Check sheet for the modelled part. Datum: model origin and axes. Units: mm. A direction names the side the tool comes from. Coordinates: 2 decimals unless noted, no trailing zeros. Loops run counter-clockwise (first coordinate to the right, second up) from the corner with the lowest first, then second, coordinate; pieces in that order, holes last. Notation, with made-up numbers: (74, -22) -> (123, -22) arc R16 cw to (123, -18) -> close; hole circle Ø4 at (-16.5, -9.75). An arc over 180 degrees is marked (long way). Use one line per item in the form item = value.
from build123d import *

# Parameters (mm, degrees)
ESBO_O1_R                = 2
ESBO_O1_R_2              = 12
ESBO_O1_W                = 46
ESBO_O1_H                = 6
ESBO_O1_H_2              = 3
RESSALTO_EXTRUS_O1_DEPTH = 3
ESBO_O1_3_W              = 46
ESBO_O1_3_H              = 3
RESSALTO_EXTRUS_O2_DEPTH = 15
ESBO_O2_R                = 2.25
ESBO_O2_R_2              = 1.5
CORTE_EXTRUS_O1_DEPTH    = 1.5
ESBO_O2_4_R              = 1.5
CORTE_EXTRUS_O3_DEPTH    = 61.580524923
RESSALTO_EXTRUS_O3_DEPTH = 2
RESSALTO_EXTRUS_O4_DEPTH = 2
CORTE_EXTRUS_O4_START    = -2
ESBO_O7_R                = 1.5
CORTE_EXTRUS_O4_DEPTH    = 2


with BuildPart() as part:
    # Esboço1 → Ressalto-extrusão1 (new body)
    # profile 1 of 4: a face of its own
    with BuildSketch(Plane.XY):
        Polygon((-23, -2), (-23, -23), (23, -23), (23, -2), (21, -2), (21, 19), (-21, 19), (-21, -2), align=None)
        with Locations((-15.731654435, -15.268345565)):
            Circle(ESBO_O1_R, mode=Mode.SUBTRACT)
        with Locations((15.26769418, -15.067384206)):
            Circle(ESBO_O1_R, mode=Mode.SUBTRACT)
        with Locations((-15.731654435, 15.731654435)):
            Circle(ESBO_O1_R, mode=Mode.SUBTRACT)
        Circle(ESBO_O1_R_2, mode=Mode.SUBTRACT)
        with Locations((15.404994987, 15.932311736)):
            Circle(ESBO_O1_R, mode=Mode.SUBTRACT)
    # profile 2 of 4: a face of its own
    with BuildSketch(Plane.XY):
        Polygon((23, -23), (-23, -23), (-23, -25), (-23, -26), (23, -26), (23, -25), align=None)
    # profile 3 of 4: a face of its own
    with BuildSketch(Plane.XY):
        with Locations((0, -29)):
            Rectangle(ESBO_O1_W, ESBO_O1_H)
    # profile 4 of 4: a face of its own
    with BuildSketch(Plane.XY):
        with Locations((0, -33.5)):
            Rectangle(ESBO_O1_W, ESBO_O1_H_2)
    extrude(amount=RESSALTO_EXTRUS_O1_DEPTH)

    # Esboço1<3> → Ressalto-extrusão2 (add)
    with BuildSketch(Plane.XY):
        Polygon((23, -23), (-23, -23), (-23, -25), (-23, -26), (23, -26), (23, -25), align=None)
        with Locations((0, -33.5)):
            Rectangle(ESBO_O1_3_W, ESBO_O1_3_H)
    extrude(amount=-RESSALTO_EXTRUS_O2_DEPTH)

    # Esboço2 → Corte-extrusão1 (cut)
    # profile 1 of 2: a face of its own
    with BuildSketch(Plane.XZ.offset(35)):
        with Locations(Location((-18, -9.5, 0), (0, 0, 270))):
            Circle(ESBO_O2_R)
        with Locations(Location((-18, -9.5, 0), (0, 0, 270))):
            Circle(ESBO_O2_R_2, mode=Mode.SUBTRACT)
    # profile 2 of 2: a face of its own
    with BuildSketch(Plane.XZ.offset(35)):
        with Locations(Location((18, -9.5, 0), (0, 0, 270))):
            Circle(ESBO_O2_R)
        with Locations(Location((18, -9.5, 0), (0, 0, 270))):
            Circle(ESBO_O2_R_2, mode=Mode.SUBTRACT)
    extrude(amount=-CORTE_EXTRUS_O1_DEPTH, mode=Mode.SUBTRACT)

    # Esboço2<4> → Corte-extrusão3 (cut, through all)
    with BuildSketch(Plane.XZ.offset(35)):
        with Locations(Location((-18, -9.5, 0), (0, 0, 270))):
            Circle(ESBO_O2_4_R)
        with Locations(Location((18, -9.5, 0), (0, 0, 270))):
            Circle(ESBO_O2_4_R)
    extrude(amount=-CORTE_EXTRUS_O3_DEPTH, mode=Mode.SUBTRACT)

    # Esboço5 → Ressalto-extrusão3 (add)
    with BuildSketch(Plane(origin=(23, 0, 0), x_dir=(0, 0, -1), z_dir=(1, 0, 0))):
        Polygon((15, -23), (0, -6.455375179), (0, -23), align=None)
    extrude(amount=-RESSALTO_EXTRUS_O3_DEPTH)

    # Esboço6 → Ressalto-extrusão4 (add)
    with BuildSketch(Plane.ZY.offset(23)):
        Polygon((-15, -23), (0, -23), (0, -6.455375179), align=None)
    extrude(amount=-RESSALTO_EXTRUS_O4_DEPTH)

    # Esboço7 → Corte-extrusão4 (cut)
    # profile 1 of 2: a face of its own
    with BuildSketch(Plane(origin=(0, -23, 0), x_dir=(1, 0, 0), z_dir=(0, 1, 0)).offset(CORTE_EXTRUS_O4_START)):
        Polygon((-20.632829264, 7.724741314), (-17.778995512, 6.332273631), (-15.146166248, 8.107532317), (-15.367170736, 11.275258686), (-18.221004488, 12.667726369), (-20.853833752, 10.892467683), align=None)
        with Locations((-18, 9.5)):
            Circle(ESBO_O7_R, mode=Mode.SUBTRACT)
    # profile 2 of 2: a face of its own
    with BuildSketch(Plane(origin=(0, -23, 0), x_dir=(1, 0, 0), z_dir=(0, 1, 0)).offset(CORTE_EXTRUS_O4_START)):
        Polygon((17.778995512, 6.332273631), (15.146166248, 8.107532317), (15.367170736, 11.275258686), (18.221004488, 12.667726369), (20.853833752, 10.892467683), (20.632829264, 7.724741314), align=None)
        with Locations((18, 9.5)):
            Circle(ESBO_O7_R, mode=Mode.SUBTRACT)
    extrude(amount=CORTE_EXTRUS_O4_DEPTH, mode=Mode.SUBTRACT)


solid = part.part
(1) Mould release check, pull along X, two halves, no side actions. Record for faces 6 (the flat face through (0, -14, 3)), 7 (the flat face through (-21, -18, -4)), 8 (the flat face through (21, 8, 1)): +X half, -X half, draft (parallel to the pull), parting line (faces both ways), or undercut.
Established:
face_6 = draft
face_7 = undercut
face_8 = +X half
(2) Tool access check on faces 1 (the flat face through (16.77, -24.01, -11.96)), 2 (the cylindrical face through (-16.17, -17.22, 1.48)), 3 (the flat face through (21, -18, -4)), 4 (the flat face through (19, -33.5, -11)), 5 (the flat face through (0, -32, -7)). Record the directions out of +Z, -Z, +X, -X, +Y, -Y that give a thin tool (end or side, any length) a straight path to the whole face; none if there is none.
Established:
face_1 = +Y
face_2 = +Z, -Z
face_3 = -Z, +Y
face_4 = -Y
face_5 = -Z, +X, -X
(3) Section check D-D, the plane x = 7. Record the boundary of the cut face in (y, z), plus the area to 3 significant figures.
Established:
outline = (-35, -15) -> (-32, -15) -> (-32, 0) -> (-26, 0) -> (-26, -15) -> (-23, -15) -> (-23, 0) -> (-9.75, 0) -> (-9.75, 3) -> (-35, 3) -> close; (9.75, 0) -> (19, 0) -> (19, 3) -> (9.75, 3) -> close
area = 194 mm²
(4) Scan lines: line 1 along X through (y, z) = (-25.45, -9.5); line 2 along X through (y, z) = (-18, -5.25); line 3 along Y through (x, z) = (16.5, -4.25). Record each from-to range of solid material in increasing order.
Established:
line_1 = -23 to -19.5, -16.5 to 16.5, 19.5 to 23
line_2 = -23 to -21, 21 to 23
line_3 = -35 to -32, -26 to -23
(5) Section check C-C, the plane z = -2.5. Record the boundary of the cut face in (x, y), plus the area to 3 significant figures.
Established:
outline = (-23, -35) -> (23, -35) -> (23, -32) -> (-23, -32) -> close; (-23, -26) -> (23, -26) -> (23, -9.21) -> (21, -9.21) -> (21, -23) -> (-21, -23) -> (-21, -9.21) -> (-23, -9.21) -> close
area = 331 mm²
(6) Go/stop test with flat-tipped pins: P1, Ø4, axis at x = 18, z = -9.5, coming from the -Y side; P2, Ø6.5, axis at x = -17.5, z = -10, coming from the +Y side; P3, Ø3.5, axis at x = 18, z = -9.5, coming from the +Y side; P4, Ø12, axis at x = 3.5, y = -29.5, coming from the -Z side. Record where each tip stops, or that it passes through.
Established:
P1 = -33.5
P2 = -23
P3 = -25
P4 = -15
(7) Section check B-B, the plane y = 0. Record the boundary of the cut face in (x, z), plus the area to 3 significant figures.
Established:
outline = (-21, 0) -> (-12, 0) -> (-12, 3) -> (-21, 3) -> close; (12, 0) -> (21, 0) -> (21, 3) -> (12, 3) -> close
area = 54.0 mm²
(8) Section check A-A, the plane x = 0. Record the boundary of the cut face in (y, z).
Established:
outline = (-35, -15) -> (-32, -15) -> (-32, 0) -> (-26, 0) -> (-26, -15) -> (-23, -15) -> (-23, 0) -> (-12, 0) -> (-12, 3) -> (-35, 3) -> close; (12, 0) -> (19, 0) -> (19, 3) -> (12, 3) -> close
